Autodesk Inventor part; units mm, degrees
ref_plane "YZ Plane" through (0, 0, 0) normal (1, 0, 0) x (0, 1, 0)
ref_plane "XZ Plane" through (0, 0, 0) normal (0, 1, 0) x (-1, 0, 0)
ref_plane "XY Plane" through (0, 0, 0) normal (0, 0, 1) x (1, 0, 0)
sketch "Sketch1" plane through (0, 0, 0) normal (0, 1, 0) x (-1, 0, 0)
  line L0 (-22.0113, 1.5875) -> (-22.0113, 7.9375)
  line L1 (-22.0113, 7.9375) -> (-9.3113, 7.9375)
  arc A0 (-3.8366, -1.5875) -> (-3.8366, 1.5875) centre (26.2841, 0) ccw
  line L2 (-22.0113, 1.5875) -> (-8.3646, 1.5875)
  line L3 (-8.3646, -1.5875) -> (-22.0113, -1.5875)
  line L4 (-22.0113, -1.5875) -> (-22.0113, -7.9375)
  line L5 (-22.0113, -7.9375) -> (-9.3113, -7.9375)
  line L6 (61.4879, 9.525) -> (100.7583, 9.525)
  line L7 (100.7583, 9.525) -> (100.7583, 3.175)
  line L8 (100.7583, 3.175) -> (62.6583, 3.175)
  line L9 (62.6583, -3.175) -> (100.7583, -3.175)
  line L10 (100.7583, -3.175) -> (100.7583, -9.525)
  line L11 (100.7583, -9.525) -> (61.4879, -9.525)
  line L12 (-8.3646, 1.5875) -> (-3.8366, 1.5875)
  line L13 (-8.3646, -1.5875) -> (-3.8366, -1.5875)
  arc A1 (61.4879, 9.525) -> (-9.3113, 7.9375) centre (26.2841, 0) ccw
  arc A2 (-9.3113, -7.9375) -> (61.4879, -9.525) centre (26.2841, 0) ccw
  arc A3 (62.6583, -3.175) -> (62.6583, 3.175) centre (26.2841, 0) ccw
  point P0 (0, 0)
  dimension "d0" = 60.325
  dimension "d2" = 6.35
  dimension "d3" = 6.35
  dimension "d4" = 3.175
  dimension "d5" = 1.5875
  dimension "d6" = 6.35
  dimension "d7" = 6.35
  dimension "d8" = 6.35
  dimension "d9" = 3.175
  dimension "d10" = 6.35
  dimension "d11" = 38.1
  dimension "d12" = 12.7
extrude "Extrusion1" add sketch "Sketch1" along normal blind 19.05
sketch "Sketch2" plane through (9.3113, 0, 7.9375) normal (0, 0, 1) x (1, 0, 0)
  circle A0 centre (6.35, 9.525) radius 2.1844
  line L0 (0, 19.05) -> (12.7, 19.05)
  line L1 (12.7, 0) -> (12.7, 19.05)
  circle A1 centre (-103.7196, 9.525) radius 2.1844
  line L2 (-110.0696, 0) -> (-110.0696, 19.05)
  line L3 (-110.0696, 19.05) -> (-70.7992, 19.05)
  point P0 (-9.3113, 0)
  dimension "d15" = 9.525
  dimension "d16" = 6.35
  dimension "d17" = 4.3688
  dimension "d18" = 6.35
  dimension "d19" = 9.525
  dimension "d20" = 4.3688
extrude "Extrusion2" cut sketch "Sketch2" along normal mid plane 50.8
fillet "Fillet1" radius 3.175 28 edges at (-81.1231, 19.05, 9.525) (-100.7583, 9.525, 9.525) (-81.1231, 0, 9.525) (-81.1231, 19.05, -9.525) (-100.7583, 9.525, -9.525) (-81.1231, 0, -9.525) (-61.4879, 9.525, -9.525) (-61.4879, 9.525, 9.525) (-62.6583, 9.525, -3.175) (-62.6583, 9.525, 3.175) (-25.4665, 19.05, -36.4605) (-25.4665, 0, -36.4605) (-25.4665, 19.05, 36.4605) (-25.4665, 0, 36.4605) (15.6613, 19.05, 7.9375) (22.0113, 9.525, 7.9375) (15.6613, 0, 7.9375) (15.6613, 19.05, -7.9375) (22.0113, 9.525, -7.9375) (15.6613, 0, -7.9375) (22.0113, 19.05, -4.7625) (22.0113, 19.05, 4.7625) (22.0113, 0, -4.7625) (22.0113, 0, 4.7625) (-100.7583, 19.05, -6.35) (-100.7583, 19.05, 6.35) (-100.7583, 0, -6.35) (-100.7583, 0, 6.35)
properties part number "Clamp"
Read the model definition and answer for the solid it produces. Units are mm, in the model's axes. A direction names the side the tool comes from. Coordinates: 2 decimals unless noted, no trailing zeros. Answer as a JSON object with one key per item and string values.
Q1. A tool of negligible diameter and unlimited length cuts with its end or side. For faces 1 (the cylindrical face through (-80.948, 18.095, 8.62)), 2 (the cylindrical face through (-80.475, 18.095, -8.62)), 3 (the flat face through (-81, 9, -9.525)), 4 (the cylindrical face through (-80.948, 0.905, 8.57)), 5 (the cylindrical face through (14.02, 18.145, -6.983)), from which of +Z, -Z, +X, -X, +Y, -Y can it reach the whole face along a straight path? Write none if from no direction.
The answers:
{"face 1": "+Z, -X, +Y", "face 2": "-Z, -X, +Y", "face 3": "-Z, -X, +Y, -Y", "face 4": "+Z, -X, -Y", "face 5": "-Z, +X, +Y"}
Q2. Determine the mould class of faces 6 (the cylindrical face through (14.02, 0.95, -7.03)), 7 (the cylindrical face through (-99.85, 18.1, -4.78)), 8 (the flat face through (13, 9, 1.588)) for opening direction Z: pulls with the +Z half, pulls with the -Z half, needs draft (parallel to the pull), parting line crosses it, or undercut.
The answers:
{"face 6": "pulls with the -Z half", "face 7": "needs draft", "face 8": "undercut"}
Q3. Flat-ended cylindrical pins translate along their axes: pin 1 Ø7 at (x, y) = (-94.41, 9.52) entering from -Z (3 decimals); pin 2 Ø4 at (x, y) = (-94.41, 9.52) entering from -Z; pin 3 Ø1 at (y, z) = (12.5, -8.5) entering from +X; pin 4 Ø5 at (x, y) = (15.66, 9.52) entering from +Z. Find the tip coordinate at first contact, or state that the pin passes through.
The answers:
{"pin 1": "stops at z = -9.525", "pin 2": "passes through", "pin 3": "stops at x = 9.3", "pin 4": "stops at z = 7.94"}
Q4. Consider line 1 (Z direction, x = -90.5, y = 12.5) (3 decimals); line 2 (Z direction, x = -88, y = 1.25) (3 decimals); line 3 (X direction, y = 16.5, z = 18). Determine where each line is inside the solid, lowest interval first. Write a range as [from, to].
The answers:
{"line 1": "z = [-9.525, -3.175], [3.175, 9.525]", "line 2": "z = [-8.875, -3.175], [3.175, 8.875]", "line 3": "x = [-57.93, -50.49], [-2.08, 5.36]"}
